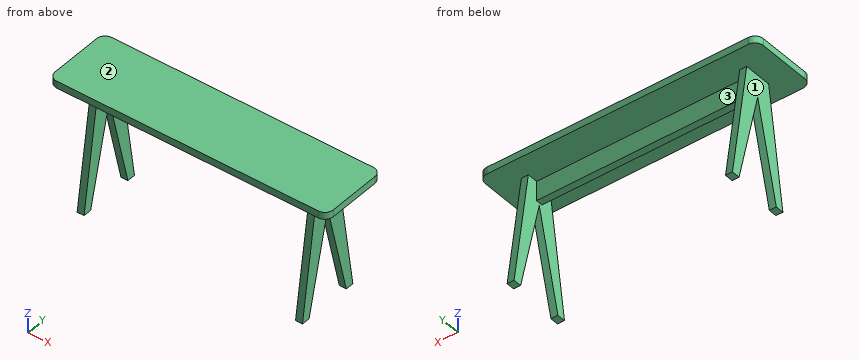
from build123d import *

# Parameters (mm, degrees)
F0_W     = 1000
F0_H     = 250
F1_DEPTH = 25
F2_W     = 380
F2_H     = 70
F3_DEPTH = 12.5
F5_START = 380
F5_DEPTH = 25
F6_START = -380
F6_DEPTH = 25
F7_R     = 30


with BuildPart() as f1:
    # F0 (on Top) → F1 (new body)
    with BuildSketch(Plane.XY):
        Rectangle(F0_W, F0_H)
    extrude(amount=F1_DEPTH)

    # F2 (on Front) → F3 (join, symmetric)
    with BuildSketch(Plane.XZ):
        with Locations((-190, -35)):
            Rectangle(F2_W, F2_H)
        with Locations((190, -35)):
            Rectangle(F2_W, F2_H)
    extrude(amount=F3_DEPTH, both=True)

    # F4 (on Right) → F5 (join)
    with BuildSketch(Plane.YZ.offset(F5_START)):
        Polygon((50, 0), (0, 0), (0, -80), (85, -425), (115, -425), align=None)
        Polygon((0, -80), (0, 0), (-50, 0), (-115, -425), (-85, -425), align=None)
    extrude(amount=F5_DEPTH)

    # F4 (on Right) → F6 (join)
    with BuildSketch(Plane.YZ.offset(F6_START)):
        Polygon((0, -80), (0, 0), (-50, 0), (-115, -425), (-85, -425), align=None)
        Polygon((50, 0), (0, 0), (0, -80), (85, -425), (115, -425), align=None)
    extrude(amount=-F6_DEPTH)

    # F7
    f7_edges = [f1.edges().sort_by_distance(p)[0] for p in [
        (500, 125, 12.5),
        (500, -125, 12.5),
        (-500, 125, 12.5),
        (-500, -125, 12.5),
    ]]
    fillet(f7_edges, radius=F7_R)


solid = f1.part
Input: part model. Units: mm. Frame: model coordinates. Face numbers are marked on the shaded views. Coordinates: 2 decimals unless noted, no trailing zeros. Loops run counter-clockwise (first coordinate to the right, second up) from the corner with the lowest first, then second, coordinate; pieces in that order, holes last.
(1) Material intervals for probe 1 along X at (y, z) = (34.5, -145); probe 2 along Z at (x, y) = (-167, -2.5); probe 3 along Z at (x, y) = (416.5, 110), sorted ascending.
(2) First-contact query: pin 1 Ø4 at (x, y) = (376, 78) entering from -Z; pin 2 Ø3 at (x, z) = (-389, -152) entering from +Y; pin 3 Ø6 at (x, z) = (-258.5, -56) entering from +Y. Flat tips, straight axial feed; report the tip coordinate or a pass-through.
(3) Section B-B on x = 124. Return the cut outline in (y, z).
(4) Section D-D on y = -63.5. Return the cut outline in (x, z), then the cut area to 3 significant figures.
(5) Section C-C on z = -375. Return the cut outline in (x, y).
(6) Pull-direction query (X, two-part tool) for the marked faces 1, 2 and 3; classes: released by +X, released by -X, zero draft, split by the parting line, or undercut.
(7) Section A-A on z = -34. Return the cut outline in (x, y).
Data:
1. probe 1: x = -405 to -380, 380 to 405
1. probe 2: z = -70 to 25
1. probe 3: z = 0 to 25
2. pin 1: stops at z = 0
2. pin 2: stops at y = 73.48
2. pin 3: stops at y = 12.5
3. outline: (-125, 0) - (-12.5, 0) - (-12.5, -70) - (12.5, -70) - (12.5, 0) - (125, 0) - (125, 25) - (-125, 25) - close
4. outline: (-500, 0) - (500, 0) - (500, 25) - (-500, 25) - close; (-405, -337.74) - (-380, -337.74) - (-380, -88.27) - (-405, -88.27) - close; (380, -337.74) - (405, -337.74) - (405, -88.27) - (380, -88.27) - close
4. area: 37,500 mm2
5. outline: (-405, -107.35) - (-380, -107.35) - (-380, -72.68) - (-405, -72.68) - close; (-405, 72.68) - (-380, 72.68) - (-380, 107.35) - (-405, 107.35) - close; (380, -107.35) - (405, -107.35) - (405, -72.68) - (380, -72.68) - close; (380, 72.68) - (405, 72.68) - (405, 107.35) - (380, 107.35) - close
6. face 1: released by -X
6. face 2: zero draft
6. face 3: undercut
7. outline: (-405, -55.2) - (-380, -55.2) - (-380, -12.5) - (380, -12.5) - (380, -55.2) - (405, -55.2) - (405, 55.2) - (380, 55.2) - (380, 12.5) - (-380, 12.5) - (-380, 55.2) - (-405, 55.2) - close
